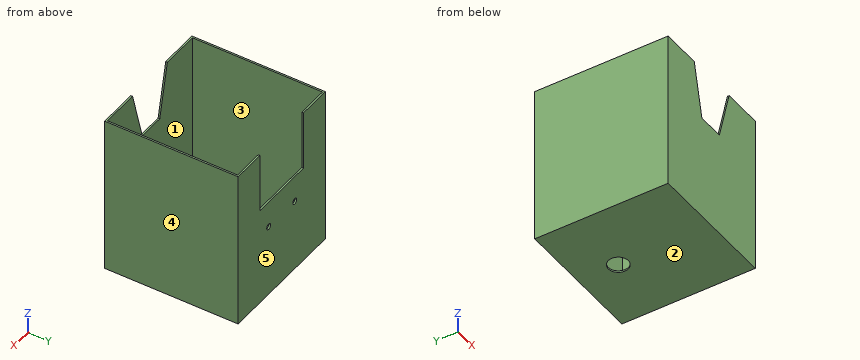
```python
from build123d import *

# Parameters (mm, degrees)
F1_DEPTH  = 254
F2_T      = -3.175
F4_DEPTH  = 25.4
F6_DEPTH  = 25.4
F8_DEPTH  = 25.4
F9_R      = 5.55625
F10_DEPTH = 25.4


with BuildPart() as f1:
    # F0 (on Front) → F1 (new body)
    with BuildSketch(Plane.XZ):
        Polygon((-127, 0), (0, 0), (127, 0), (127, 304.8), (-127, 304.8), align=None)
    extrude(amount=-F1_DEPTH)

    # F2
    f2_openings = [f1.faces().sort_by_distance(p)[0] for p in [
        (0, 127, 304.8),
    ]]
    offset(amount=F2_T, openings=f2_openings)

    # F3 (on face) → F4 (cut)
    with BuildSketch(Plane.XZ):
        Polygon((50.8, 304.8), (-50.8, 304.8), (-28.575, 203.2), (22.225, 203.2), align=None)
    extrude(amount=-F4_DEPTH, mode=Mode.SUBTRACT)

    # F5 (on face) → F6 (cut)
    with BuildSketch(Plane(origin=(0, 254, 0), x_dir=(-1, 0, 0), z_dir=(0, 1, 0))):
        Polygon((-16.939813, 304.8), (-63.5, 304.8), (-63.5, 190.5), (-16.939813, 190.5), (63.5, 190.5), (63.5, 304.8), align=None)
    extrude(amount=-F6_DEPTH, mode=Mode.SUBTRACT)

    # F7 (on face) → F8 (cut)
    with BuildSketch(Plane(origin=(0, 0, 0), x_dir=(1, 0, 0), z_dir=(0, 0, -1))):
        with BuildLine():
            ThreePointArc((0, -158.75), (-13.470384, -191.270384), (19.05, -177.8))
            ThreePointArc((19.05, -177.8), (13.470384, -164.329616), (0, -158.75))
        make_face()
    extrude(amount=-F8_DEPTH, mode=Mode.SUBTRACT)

    # F9 (on face) → F10 (cut)
    with BuildSketch(Plane(origin=(0, 254, 0), x_dir=(-1, 0, 0), z_dir=(0, 1, 0))):
        with BuildLine():
            ThreePointArc((43.65625, 139.7), (38.1, 145.25625), (32.54375, 139.7))
            ThreePointArc((32.54375, 139.7), (38.1, 134.14375), (43.65625, 139.7))
        make_face()
        with Locations((-38.1, 139.7)):
            Circle(F9_R)
    extrude(amount=-F10_DEPTH, mode=Mode.SUBTRACT)


solid = f1.part
```
Build history of the part. All positions in model axes, mm. Face numbers are marked on the shaded views. A direction names the side the tool comes from. Give positions to 0.01 mm unless a question says otherwise; leave off trailing zeros. Loops run counter-clockwise (first coordinate to the right, second up) from the corner with the lowest first, then second, coordinate; pieces in that order, holes last.
1) Band-saw the part on B-B on y = 62. List the corners of the cut face in (x, z) (3 decimals), then the cut area to 3 significant figures.
Values follow:
outline: (-127, 0) - (127, 0) - (127, 304.8) - (123.825, 304.8) - (123.825, 3.175) - (-123.825, 3.175) - (-123.825, 304.8) - (-127, 304.8) - close
area: 2,720 mm2
2) 3-axis set-ups, long thin cutter, end or side, ignore diameter. For the marked faces 1 and 2: which of +Z, -Z, +X, -X, +Y, -Y reach the whole face in a straight line?
Values follow:
face 1: +Z
face 2: -Z, +X, -X, +Y, -Y
3) Drop flat-ended pins along their axis: P1, Ø1, axis at x = 21, y = 253, coming from the +Z side; P2, Ø8, axis at x = 18, y = 131, coming from the +Z side (3 decimals); P3, Ø1, axis at x = 2, y = 1.5, coming from the +Z side. Give the stop position or say it passes through.
Values follow:
P1: stops at z = 190.5
P2: stops at z = 3.175
P3: stops at z = 203.2
4) Band-saw the part on D-D on z = 63. List the corners of the cut face in (x, y) (3 decimals).
Values follow:
outline: (-127, 0) - (127, 0) - (127, 254) - (-127, 254) - close; hole (-123.825, 3.175) - (123.825, 3.175) - (123.825, 250.825) - (-123.825, 250.825) - close
5) Probe line 1 along X through (y, z) = (251, 139); line 2 along X through (y, z) = (177.8, 1.65); line 3 along Y through (x, z) = (0, 68.5) (3 decimals). List the from-to ranges inside material, lowest first.
Values follow:
line 1: x = -127 to -43.61, -32.59 to 32.59, 43.61 to 127
line 2: x = -127 to -19.05, 19.05 to 127
line 3: y = 0 to 3.175, 250.825 to 254
6) Band-saw the part on A-A on z = 139.7. List the corners of the cut face in (x, y) (3 decimals).
Values follow:
outline: (-127, 0) - (127, 0) - (127, 254) - (43.656, 254) - (43.656, 250.825) - (123.825, 250.825) - (123.825, 3.175) - (-123.825, 3.175) - (-123.825, 250.825) - (-43.656, 250.825) - (-43.656, 254) - (-127, 254) - close; (-32.544, 250.825) - (32.544, 250.825) - (32.544, 254) - (-32.544, 254) - close
7) Band-saw the part on C-C on x = 38.1. List the corners of the cut face in (y, z) (3 decimals), then the cut area to 3 significant figures.
Values follow:
outline: (0, 0) - (254, 0) - (254, 134.144) - (250.825, 134.144) - (250.825, 3.175) - (3.175, 3.175) - (3.175, 259.644) - (0, 259.644) - close; (250.825, 145.256) - (254, 145.256) - (254, 190.5) - (250.825, 190.5) - close
area: 2,180 mm2
8) Two-plate mould, pull along Y, no slides. Class the marked faces 3, 4 and 5: released by +Y, released by -Y, zero draft, split by the parting line, or undercut.
Values follow:
face 3: undercut
face 4: zero draft
face 5: released by +Y
